Autodesk Inventor part; units mm, degrees
ref_plane "YZ Plane" through (0, 0, 0) normal (1, 0, 0) x (0, 1, 0)
ref_plane "XZ Plane" through (0, 0, 0) normal (0, 1, 0) x (-1, 0, 0)
ref_plane "XY Plane" through (0, 0, 0) normal (0, 0, 1) x (1, 0, 0)
sketch "スケッチ1" plane through (0, 0, 0) normal (0, 0, 1) x (1, 0, 0)
  line L0 (35.3, 43.5) -> (-35.3, 43.5)
  line L1 (-35.3, 43.5) -> (-35.3, -43.5)
  line L2 (-35.3, -43.5) -> (35.3, -43.5)
  line L3 (35.3, -43.5) -> (35.3, 43.5)
  line L4 (35.3, 43.5) -> (-35.3, -43.5) construction
  line L5 (-35.3, 43.5) -> (35.3, -43.5) construction
  line L6 (35.3, 24) -> (29.7, 24)
  line L7 (29.7, 24) -> (29.7, -24)
  line L8 (29.7, -24) -> (35.3, -24)
  line L9 (35.3, 0) -> (-35.3, 0) construction
  line L10 (10.7, -39.5) -> (-31.3, -39.5) construction
  line L11 (-31.3, -39.5) -> (-31.3, 39.5) construction
  line L12 (-31.3, 39.5) -> (10.7, 39.5) construction
  line L13 (10.7, 39.5) -> (10.7, -39.5) construction
  line L14 (10.7, -39.5) -> (-31.3, 39.5) construction
  line L15 (-31.3, -39.5) -> (10.7, 39.5) construction
  circle A0 centre (-31.3, 39.5) radius 1.6
  circle A1 centre (10.7, 39.5) radius 1.6
  circle A2 centre (-31.3, -39.5) radius 1.6
  circle A3 centre (10.7, -39.5) radius 1.6
  point P0 (0, 0)
  point P1 (-10.3, 0)
  dimension "d0" = 70.6
  dimension "d1" = 87
  dimension "d2" = 19.5
  dimension "d3" = 48
  dimension "d4" = 65
  dimension "d5" = 4
  dimension "d6" = 4
  dimension "d7" = 46
  dimension "d8" = 3.2
  dimension "d9" = 3.2
extrude "押し出し1" add sketch "スケッチ1" along normal blind 1.6 contours L3 L6 L7 L8 L2 L1 L0
equation "\"d9\" = d8"
properties part number "EN715_with_JetsonXavierNX_and_Fan"
Check sheet for the modelled part. Datum: model origin and axes. Units: mm. Give positions to 0.01 mm unless a question says otherwise; leave off trailing zeros. Order: outer loops, then holes, each group sorted by start corner. A loop starts at its lowest first (then second) coordinate and runs counter-clockwise, first axis right, second up. Notation, with made-up numbers: (64.5, 14) -> (74.5, 14) arc R22 cw to (74.5, 48) -> close; hole circle Ø5 at (41.25, 64). An arc over 180 degrees is marked (long way). Return JSON: item names as keys, results as strings.
1. Cross-section at C-C, the plane z = 0.45. Record the cut outline in (x, y).
From the geometry:
{"outline": "(-35.3, -43.5) -> (35.3, -43.5) -> (35.3, -24) -> (29.7, -24) -> (29.7, 24) -> (35.3, 24) -> (35.3, 43.5) -> (-35.3, 43.5) -> close; hole circle Ø3.2 at (-31.3, -39.5); hole circle Ø3.2 at (-31.3, 39.5); hole circle Ø3.2 at (10.7, -39.5); hole circle Ø3.2 at (10.7, 39.5)"}
2. Cross-section at D-D, the plane y = 17. Record the cut outline in (x, z).
From the geometry:
{"outline": "(-35.3, 0) -> (29.7, 0) -> (29.7, 1.6) -> (-35.3, 1.6) -> close"}
3. Cross-section at A-A, the plane x = 10.7. Record the cut outline in (y, z).
From the geometry:
{"outline": "(-43.5, 0) -> (-41.1, 0) -> (-41.1, 1.6) -> (-43.5, 1.6) -> close; (-37.9, 0) -> (37.9, 0) -> (37.9, 1.6) -> (-37.9, 1.6) -> close; (41.1, 0) -> (43.5, 0) -> (43.5, 1.6) -> (41.1, 1.6) -> close"}
4. Material ranges on probe 1 along Y at (x, z) = (10.7, 0.65); probe 2 along Y at (x, z) = (32, 1.55); probe 3 along X at (y, z) = (1, 0.6), recorded low to high. Write a range as [from, to].
From the geometry:
{"probe 1": "[-43.5, -41.1], [-37.9, 37.9], [41.1, 43.5]", "probe 2": "[-43.5, -24], [24, 43.5]", "probe 3": "[-35.3, 29.7]"}
5. Mould release check, pull along Y, two halves, no side actions. Record for faces 1 (the cylindrical face through (-32.57, 40.47, 0.79)), 2 (the flat face through (0, 1, 0)): +Y half, -Y half, draft (parallel to the pull), parting line (faces both ways), or undercut.
From the geometry:
{"face 1": "undercut", "face 2": "draft"}
6. Cross-section at B-B, the plane y = -39.5. Record the cut outline in (x, z).
From the geometry:
{"outline": "(-35.3, 0) -> (-32.9, 0) -> (-32.9, 1.6) -> (-35.3, 1.6) -> close; (-29.7, 0) -> (9.1, 0) -> (9.1, 1.6) -> (-29.7, 1.6) -> close; (12.3, 0) -> (35.3, 0) -> (35.3, 1.6) -> (12.3, 1.6) -> close"}
